from build123d import *

# Parameters (mm, degrees)
F0_W        = 38.1
F0_H        = 44.45
F1_DEPTH    = 31.75
F2_R        = 6.35
F3_DEPTH    = 6.35
F4_R        = 3.175
F5_DEPTH    = 2.54
F6_T1_DEPTH = 57.15


# Not quite as in the source:
# - a fillet or chamfer that OpenCascade refuses, or shapes differently, is made with other operations: its cross-section is extruded or revolved along the edge and cut away or added


with BuildPart() as f1:
    # F0 (on Front) → F1 (new body)
    with BuildSketch(Plane.XZ):
        Rectangle(F0_W, F0_H)
    extrude(amount=F1_DEPTH)

    # F2 (on face) → F3 (cut)
    with BuildSketch(Plane.XZ.offset(31.75)):
        with Locations((-11.43, -14.605)):
            Circle(F2_R)
    extrude(amount=-F3_DEPTH, mode=Mode.SUBTRACT)

    # F4 (on face) → F5 (join)
    with BuildSketch(Plane.XY.offset(22.225)):
        with Locations((11.43, -24.13)):
            Circle(F4_R)
    extrude(amount=F5_DEPTH)

    # F6: fillet of radius 2.54 on 4 edges, made by hand

    # F6_s2 → F6_t1 (cut)
    with BuildSketch(Plane.XY.offset(-28.575)):
        with BuildLine():
            ThreePointArc((-16.51, -31.75), (-18.3060512242, -31.0060512242), (-19.05, -29.21))
            Line((-19.05, -29.21), (-19.05, -31.75))
            Line((-19.05, -31.75), (-16.51, -31.75))
        make_face()
        with BuildLine():
            ThreePointArc((19.05, -29.21), (18.3060512242, -31.0060512242), (16.51, -31.75))
            Line((16.51, -31.75), (19.05, -31.75))
            Line((19.05, -31.75), (19.05, -29.21))
        make_face()
        with BuildLine():
            ThreePointArc((-16.51, 0), (-18.3060512242, -0.7439487758), (-19.05, -2.54))
            Line((-19.05, -2.54), (-19.05, 0))
            Line((-19.05, 0), (-16.51, 0))
        make_face()
        with BuildLine():
            ThreePointArc((19.05, -2.54), (18.3060512242, -0.7439487758), (16.51, 0))
            Line((16.51, 0), (19.05, 0))
            Line((19.05, 0), (19.05, -2.54))
        make_face()
    extrude(amount=F6_T1_DEPTH, mode=Mode.SUBTRACT)


solid = f1.part
Verification items for the finished model (mm, model axes). A direction names the side the tool comes from. Give positions to 0.01 mm unless a question says otherwise; leave off trailing zeros. Loops run counter-clockwise (first coordinate to the right, second up) from the corner with the lowest first, then second, coordinate; pieces in that order, holes last. Notation, with made-up numbers: (19, -37) - (31, -37) arc R30 ccw to (31, -11) - close; hole circle Ø10 at (-17, -21). An arc over 180 degrees is marked (long way). Write item = value, one per line. Start each with the question number.
Q1. Cross-section at B-B, the plane x = 11.43. Enter the section's corners in (y, z) (3 decimals), and give its area (3 significant figures).
Q2. Cross-section at C-C, the plane y = -7. Enter the section's corners in (x, z) (3 decimals), and give its area (3 significant figures).
Q3. Tool access check on faces 4 (the face through (-5.564, -28.619, -17.037)), 5 (the face through (-18.286, -0.724, -0.311)), 6 (the face through (11.02, -20.98, 23.48)). Record the directions out of +Z, -Z, +X, -X, +Y, -Y that give a thin tool (end or side, any length) a straight path to the whole face; none if there is none.
Q4. Cross-section at A-A, the plane y = -24.13. Enter the section's corners in (x, z) (3 decimals).
Q5. Cross-section at D-D, the plane x = -4. Enter the section's corners in (y, z) (3 decimals).
Q6. Thickness scan on line 1 (Z direction, x = 17, y = -17) (3 decimals); line 2 (Z direction, x = -7, y = -26) (3 decimals); line 3 (Z direction, x = -11, y = -29) (3 decimals). Record the ranges inside material, lowest first.
Q7. Mould release check, pull along Z, two halves, no side actions. Record for faces 1 (the face through (-12, -25.4, -15)), 2 (the face through (0, -16, 22.225)), 3 (the face through (18.326, -30.986, -0.311)): released by +Z, released by -Z, zero draft, split by the parting line, or undercut.
Q8. Depth check by flat-ended pin: P1, Ø10, axis at x = -11.5, z = -16, coming from the -Y side; P2, Ø2, axis at x = -4, y = -23, coming from the +Z side (3 decimals). Enter the tip coordinate at first touch or a pass-through.
Answer key:
q1.outline = (-31.75, -22.225) - (0, -22.225) - (0, 22.225) - (-20.955, 22.225) - (-20.955, 24.765) - (-27.305, 24.765) - (-27.305, 22.225) - (-31.75, 22.225) - close
q1.area = 1,430 mm^2
q2.outline = (-19.05, -22.225) - (19.05, -22.225) - (19.05, 22.225) - (-19.05, 22.225) - close
q2.area = 1,690 mm^2
q3.face_4 = -Y
q3.face_5 = +Z, -Z, -X, +Y
q3.face_6 = +Z
q4.outline = (-19.05, -22.225) - (19.05, -22.225) - (19.05, 22.225) - (14.605, 22.225) - (14.605, 24.765) - (8.255, 24.765) - (8.255, 22.225) - (-19.05, 22.225) - close
q5.outline = (-31.75, -22.225) - (0, -22.225) - (0, 22.225) - (-31.75, 22.225) - close
q6.line_1 = -22.225 to 22.225
q6.line_2 = -22.225 to -19.154, -10.056 to 22.225
q6.line_3 = -22.225 to -20.94, -8.27 to 22.225
q7.face_1 = undercut
q7.face_2 = released by +Z
q7.face_3 = zero draft
q8.P1 = -31.75
q8.P2 = 22.225
